Input: part model. Units: mm. Frame: model coordinates. A direction names the side the tool comes from. Round coordinates to 2 decimals unless told otherwise and drop trailing zeros. Loops run counter-clockwise (first coordinate to the right, second up) from the corner with the lowest first, then second, coordinate; pieces in that order, holes last. Notation, with made-up numbers: (9, -38) - (55, -38) arc R29 cw to (55, -5) - close; hole circle Ø4 at (47, 6). An arc over 180 degrees is marked (long way). Use CSV: the item, a comma, the result in double quotes. Start each with the question number.
1. Cut plane C-C (x = -4). Give the number of separate pieces and of enclosed holes in the cut face, and give its area (3 significant figures).
2. Access query for faces 1 (the flat face through (0, 0.75, -5)), 2 (the cylindrical face through (0, 5, -6)), 3 (the flat face through (0, -4, -5)), 4 (the cylindrical face through (3.34, -1.05, -2.46)). Directions: +Z, -Z, +X, -X, +Y, -Y. A direction counts if a zero-diameter tool reaches every point of the face in a straight line with its end or side. Return the directions, or none.
3. Pin query (flat end, axial travel): P1, Ø1.6, axis at x = 0, z = -4, coming from the -Y side; P2, Ø2, axis at y = 3, z = -4.5, coming from the +X side. Return the tip coordinate at first contact, or that it passes through.
4. Pull-direction query (Z, two-part tool) for faces 5 (the flat face through (0, -0.75, -5)), 6 (the flat face through (1.5, 3.4, 0)), 7 (the flat face through (0, 2, -8)); classes: +Z half, -Z half, draft (parallel to the pull), parting line (faces both ways), or undercut.
5. Material intervals for probe 1 along Z at (x, y) = (-3.25, 4); probe 2 along Z at (x, y) = (-3.25, -2.5); probe 3 along Y at (x, z) = (3.25, -5.25), sorted ascending. Write a range as from..to.
6. Cut plane A-A (x = 0). Return loops of the section in (y, z).
7. Cut plane B-B (z = -5.5). Return loops of the section in (x, y).
```python
from build123d import *

# Parameters (mm, degrees)
SKETCH087_W     = 14
SKETCH087_H     = 10
PAD045_DEPTH    = 2
SKETCH088_R     = 3.5
PAD046_DEPTH    = 5
SKETCH089_R     = 5
PAD047_DEPTH    = 3
POCKET037_DEPTH = 14
FILLET007_R     = 0.5


with BuildPart() as part:
    # Sketch087 → Pad045 (new body)
    with BuildSketch(Plane.XY):
        Rectangle(SKETCH087_W, SKETCH087_H)
    extrude(amount=PAD045_DEPTH)

    # Sketch088 (on Face5 of Pad045) → Pad046 (join)
    with BuildSketch(Plane(origin=(0, 0, 0), x_dir=(1, 0, 0), z_dir=(0, 0, -1))):
        Circle(SKETCH088_R)
    extrude(amount=PAD046_DEPTH)

    # Sketch089 (on Face8 of Pad046) → Pad047 (join)
    with BuildSketch(Plane(origin=(0, 0, -5), x_dir=(1, 0, 0), z_dir=(0, 0, -1))):
        Circle(SKETCH089_R)
    extrude(amount=PAD047_DEPTH)

    # Sketch090 (on Face1 of Pad047) → Pocket037 (cut)
    with BuildSketch(Plane(origin=(-7, 0, 0), x_dir=(0, -1, 0), z_dir=(-1, 0, 0))):
        Polygon((-0.75, -2), (-0.75, -8), (0.75, -8), (0.75, -2), (0, -1.474844), align=None)
    extrude(amount=-POCKET037_DEPTH, mode=Mode.SUBTRACT)

    # Fillet007
    fillet007_edges = [part.edges().sort_by_distance(p)[0] for p in [
        (0, -5, -8),
        (0, -0.75, -8),
        (0, 0.75, -8),
        (0, 5, -8),
    ]]
    fillet(fillet007_edges, radius=FILLET007_R)


solid = part.part
```
Established:
1,separate pieces,"3"
1,enclosed holes,"0"
1,area,"33.2 mm2"
2,face 1,"-Z, +X, -X"
2,face 2,"-Z, +Y"
2,face 3,"-Y"
2,face 4,"none"
3,P1,"stops at y = -3.5"
3,P2,"stops at x = 4.52"
4,face 5,"draft"
4,face 6,"undercut"
4,face 7,"-Z half"
5,probe 1,"z = 0..2"
5,probe 2,"z = -8..-5, 0..2"
5,probe 3,"y = -3.8..-0.75, 0.75..3.8"
6,outline,"(-5, -7.5) arc R0.5 ccw to (-4.5, -8) - (-1.25, -8) arc R0.5 ccw to (-0.75, -7.5) - (-0.75, -2) - (0, -1.47) - (0.75, -2) - (0.75, -7.5) arc R0.5 ccw to (1.25, -8) - (4.5, -8) arc R0.5 ccw to (5, -7.5) - (5, -5) - (3.5, -5) - (3.5, 0) - (5, 0) - (5, 2) - (-5, 2) - (-5, 0) - (-3.5, 0) - (-3.5, -5) - (-5, -5) - close"
7,outline,"(-4.94, -0.75) arc R5 ccw to (4.94, -0.75) - close; (-4.94, 0.75) - (4.94, 0.75) arc R5 ccw to start"
